```python
from build123d import *

# Parameters (mm, degrees)
F0_W         = 150
F0_H         = 100
F0_R         = 14
F1_DEPTH     = 2
F2_R         = 20
F3_T1_DEPTH  = 110
F3_T3_DEPTH  = 60
F3_T6_ANGLE  = 90
F3_T8_ANGLE  = 90
F3_T10_ANGLE = 90
F3_T12_ANGLE = 90


# Not quite as in the source:
# - a fillet or chamfer that OpenCascade refuses, or shapes differently, is made with other operations: its cross-section is extruded or revolved along the edge and cut away or added


with BuildPart() as f1:
    # F0 (on Top) → F1 (new body)
    with BuildSketch(Plane.XY):
        Rectangle(F0_W, F0_H)
        with Locations((-27.0043395302, -25.9092412172)):
            Circle(F0_R, mode=Mode.SUBTRACT)
        with Locations((5.1257033043, -19.4994347856)):
            Circle(F0_R, mode=Mode.SUBTRACT)
        with Locations((38.5656639238, -17.7100679294)):
            Circle(F0_R, mode=Mode.SUBTRACT)
        with Locations((-35.8011273407, 5.9865840333)):
            Circle(F0_R, mode=Mode.SUBTRACT)
        with Locations((-2.5469161856, 12.3156928879)):
            Circle(F0_R, mode=Mode.SUBTRACT)
        with Locations((29.6401518762, 15.2098077585)):
            Circle(F0_R, mode=Mode.SUBTRACT)
    extrude(amount=F1_DEPTH)

    # F2
    f2_edges = [f1.edges().sort_by_distance(p)[0] for p in [
        (-75, -50, 1),
        (75, -50, 1),
        (-75, 50, 1),
        (75, 50, 1),
    ]]
    fillet(f2_edges, radius=F2_R)

    # F3: fillet of radius 5 on 2 edges, made by hand

    # F3_s2 → F3_t1 (cut)
    with BuildSketch(Plane.YZ.offset(-55)):
        with BuildLine():
            ThreePointArc((-50, 0), (-48.2360679775, 1.472135955), (-46, 2))
            Line((-46, 2), (-50, 2))
            Line((-50, 2), (-50, 0))
        make_face()
        with BuildLine():
            ThreePointArc((46, 2), (48.2360679775, 1.472135955), (50, 0))
            Line((50, 0), (50, 2))
            Line((50, 2), (46, 2))
        make_face()
    extrude(amount=F3_T1_DEPTH, mode=Mode.SUBTRACT)

    # F3_s4 → F3_t3 (cut)
    with BuildSketch(Plane.XZ.offset(-30)):
        with BuildLine():
            ThreePointArc((-71, 2), (-73.2360679775, 1.472135955), (-75, 0))
            Line((-75, 0), (-75, 2))
            Line((-75, 2), (-71, 2))
        make_face()
        with BuildLine():
            ThreePointArc((71, 2), (73.2360679775, 1.472135955), (75, 0))
            Line((75, 0), (75, 2))
            Line((75, 2), (71, 2))
        make_face()
    extrude(amount=F3_T3_DEPTH, mode=Mode.SUBTRACT)

    # F3_s5 → F3_t6 (revolve, cut)
    with BuildSketch(Plane.YZ.offset(-55)):
        with BuildLine():
            ThreePointArc((-50, 0), (-48.2360679775, 1.472135955), (-46, 2))
            Line((-46, 2), (-50, 2))
            Line((-50, 2), (-50, 0))
        make_face()
    revolve(axis=Axis((-55, -30, 2), (0, 0, -1)), revolution_arc=F3_T6_ANGLE, mode=Mode.SUBTRACT)

    # F3_s7 → F3_t8 (revolve, cut)
    with BuildSketch(Plane.YZ.offset(-55)):
        with BuildLine():
            ThreePointArc((46, 2), (48.2360679775, 1.472135955), (50, 0))
            Line((50, 0), (50, 2))
            Line((50, 2), (46, 2))
        make_face()
    revolve(axis=Axis((-55, 30, 2), (0, 0, 1)), revolution_arc=F3_T8_ANGLE, mode=Mode.SUBTRACT)

    # F3_s9 → F3_t10 (revolve, cut)
    with BuildSketch(Plane.XZ.offset(-30)):
        with BuildLine():
            ThreePointArc((71, 2), (73.2360679775, 1.472135955), (75, 0))
            Line((75, 0), (75, 2))
            Line((75, 2), (71, 2))
        make_face()
    revolve(axis=Axis((55, 30, 2), (0, 0, 1)), revolution_arc=F3_T10_ANGLE, mode=Mode.SUBTRACT)

    # F3_s11 → F3_t12 (revolve, cut)
    with BuildSketch(Plane.YZ.offset(55)):
        with BuildLine():
            ThreePointArc((-50, 0), (-48.2360679775, 1.472135955), (-46, 2))
            Line((-46, 2), (-50, 2))
            Line((-50, 2), (-50, 0))
        make_face()
    revolve(axis=Axis((55, -30, 2), (0, 0, 1)), revolution_arc=F3_T12_ANGLE, mode=Mode.SUBTRACT)


solid = f1.part
```
Work out the finished part from the listing and answer in its coordinate system (mm). Coordinates: 2 decimals unless noted, no trailing zeros. Order: outer loops, then holes, each group sorted by start corner. A loop starts at its lowest first (then second) coordinate and runs counter-clockwise, first axis right, second up. Notation, with made-up numbers: (6.5, 33.5) - (20.5, 33.5) arc R13 ccw to (20.5, 52.5) - close; hole circle Ø1 at (-28, -3.75). An arc over 180 degrees is marked (long way). Answer as a JSON object with one key per item and string values.
1. Find section B-B on x = 9. Determine the outline of the cut face in (y, z), plus the area to 3 significant figures.
Output values:
{"outline": "(-50, 0) - (-32.95, 0) - (-32.95, 2) - (-46, 2) arc R5 ccw to start; (-6.05, 0) - (4.4, 0) - (4.4, 2) - (-6.05, 2) - close; (20.23, 0) - (50, 0) arc R5 ccw to (46, 2) - (20.23, 2) - close", "area": "110 mm²"}
2. Find section A-A on y = 17.5. Determine the outline of the cut face in (x, z), plus the area to 3 significant figures.
Output values:
{"outline": "(-75, 0) - (-43.77, 0) - (-43.77, 2) - (-71, 2) arc R5 ccw to start; (-27.84, 0) - (-15.55, 0) - (-15.55, 2) - (-27.84, 2) - close; (10.46, 0) - (15.83, 0) - (15.83, 2) - (10.46, 2) - close; (43.45, 0) - (75, 0) arc R5 ccw to (71, 2) - (43.45, 2) - close", "area": "156 mm²"}
3. Find section D-D on x = -35. Determine the outline of the cut face in (y, z).
Output values:
{"outline": "(-50, 0) - (-37.4, 0) - (-37.4, 2) - (-46, 2) arc R5 ccw to start; (-14.42, 0) - (-7.99, 0) - (-7.99, 2) - (-14.42, 2) - close; (19.96, 0) - (50, 0) arc R5 ccw to (46, 2) - (19.96, 2) - close"}
4. The mould has two halves that part along X. Classify faces 1 (the face through (73.207, 0.42, 1.487)), 2 (the face through (11.586, -31.92, 0.986)), 3 (the face through (-0.77, -48.265, 1.458)), 4 (the face through (-22.87, 0.62, 0.99)): +X half, -X half, draft (parallel to the pull), parting line (faces both ways), or undercut.
Output values:
{"face 1": "+X half", "face 2": "undercut", "face 3": "draft", "face 4": "undercut"}
5. Find section C-C on z = 0.4. Determine the outline of the cut face in (x, y), plus the area to 3 significant figures.
Output values:
{"outline": "(-74.67, -30) arc R19.67 ccw to (-55, -49.67) - (55, -49.67) arc R19.67 ccw to (74.67, -30) - (74.67, 30) arc R19.67 ccw to (55, 49.67) - (-55, 49.67) arc R19.67 ccw to (-74.67, 30) - close; hole circle Ø28 at (-35.8, 5.99); hole circle Ø28 at (-27, -25.91); hole circle Ø28 at (-2.55, 12.32); hole circle Ø28 at (5.13, -19.5); hole circle Ø28 at (29.64, 15.21); hole circle Ø28 at (38.57, -17.71)", "area": "10,800 mm²"}
6. Consider line 1 (Y direction, x = 9, z = 1.45); line 2 (Y direction, x = -6, z = 1.6); line 3 (X direction, y = -29, z = 0.9). Determine where each line is inside the solid, lowest interval first.
Output values:
{"line 1": "y = -48.28 to -32.95, -6.05 to 4.4, 20.23 to 48.28", "line 2": "y = -47.96 to -28, -11 to -1.25, 25.88 to 47.96", "line 3": "x = -74.13 to -40.66, -13.35 to -5.16, 15.41 to 30.29, 46.84 to 74.13"}
